from build123d import *

# Parameters (mm, degrees)
SKETCH_W             = 27
SKETCH_H             = 75
PAD_DEPTH            = 8
PAD001_DEPTH         = 2
SKETCH004_R          = 2.5
PAD002_DEPTH         = 2.2
SKETCH005_R          = 1.25
POCKET_DEPTH         = 4.201
SKETCH006_R          = 1.8
POCKET001_DEPTH      = 1.5
POCKET002_DEPTH      = 3.5
SKETCH008_R          = 2.5
PAD003_DEPTH         = 10
SKETCH009_R          = 1.5
POCKET003_DEPTH      = 13
POCKET004_DEPTH      = 1.4
POCKET004_DEPTH_BACK = 2
POCKET005_DEPTH      = 2


with BuildPart() as part:
    # Sketch → Pad (new body)
    with BuildSketch(Plane.XY):
        Polygon((0, 0), (15.5, 0), (15.5, 39.5), (15.5, 79), (0, 79), (-15.5, 79), (-15.5, 39.5), (-15.5, 0), align=None)
        with Locations((0, 39.5)):
            Rectangle(SKETCH_W, SKETCH_H, mode=Mode.SUBTRACT)
    extrude(amount=PAD_DEPTH)

    # Sketch001 → Pad001 (join)
    with BuildSketch(Plane.XY):
        Polygon((-15.5, 79), (-15.5, 39.5), (-15.5, 0), (0, 0), (15.5, 0), (15.5, 39.5), (15.5, 79), (0, 79), align=None)
    extrude(amount=-PAD001_DEPTH)

    # Sketch004 → Pad002 (join)
    with BuildSketch(Plane.XY):
        with Locations((-5.5, 69.25)):
            Circle(SKETCH004_R)
        with Locations((5.5, 69.25)):
            Circle(SKETCH004_R)
    extrude(amount=PAD002_DEPTH)

    # Sketch005 (on DatumPlane) → Pocket (cut, through all)
    with BuildSketch(Plane(origin=(-3, 69.25, 2.2), x_dir=(-1, 0, 0), z_dir=(0, 0, 1))):
        with Locations((2.5, 0)):
            Circle(SKETCH005_R)
        with Locations((-8.5, 0)):
            Circle(SKETCH005_R)
    extrude(amount=-POCKET_DEPTH, mode=Mode.SUBTRACT)

    # Sketch006 (on DatumPlane) → Pocket001 (cut)
    with BuildSketch(Plane(origin=(0, 79, -2), x_dir=(1, 0, 0), z_dir=(0, 0, -1))):
        with Locations((-5.5, 9.75)):
            Circle(SKETCH006_R)
        with Locations((5.5, 9.75)):
            Circle(SKETCH006_R)
    extrude(amount=-POCKET001_DEPTH, mode=Mode.SUBTRACT)

    # Sketch007 (on DatumPlane) → Pocket002 (cut)
    with BuildSketch(Plane(origin=(0, 69.25, 3.45), x_dir=(0, 1, 0), z_dir=(0, 0, 1))):
        Polygon((9.75, 0), (9.75, 4.25), (7.75, 4.25), (7.75, -4.25), (9.75, -4.25), align=None)
    extrude(amount=POCKET002_DEPTH, mode=Mode.SUBTRACT)

    # Sketch008 (on DatumPlane) → Pad003 (join)
    with BuildSketch(Plane(origin=(0, 79, 8), x_dir=(-1, 0, 0), z_dir=(0, 0, 1))):
        with Locations((-13, 15)):
            Circle(SKETCH008_R)
        with Locations((13, 15)):
            Circle(SKETCH008_R)
        with Locations((-13, 64)):
            Circle(SKETCH008_R)
        with Locations((13, 64)):
            Circle(SKETCH008_R)
    extrude(amount=-PAD003_DEPTH)

    # Sketch009 (on DatumPlane) → Pocket003 (cut)
    with BuildSketch(Plane(origin=(0, 79, 8), x_dir=(-1, 0, 0), z_dir=(0, 0, 1))):
        with Locations((-13, 15)):
            Circle(SKETCH009_R)
        with Locations((13, 15)):
            Circle(SKETCH009_R)
        with Locations((-13, 64)):
            Circle(SKETCH009_R)
        with Locations((13, 64)):
            Circle(SKETCH009_R)
    extrude(amount=-POCKET003_DEPTH, mode=Mode.SUBTRACT)

    # Sketch010 (on DatumPlane) → Pocket004 (cut, two sides)
    with BuildSketch(Plane(origin=(0, 69.25, 3.45), x_dir=(0, 1, 0), z_dir=(0, 0, 1))) as pocket004_sk:
        Polygon((7.75, 0), (7.75, 10), (8.75, 10), (8.75, -10), (7.75, -10), align=None)
    extrude(amount=-POCKET004_DEPTH, mode=Mode.SUBTRACT)
    extrude(pocket004_sk.sketch, amount=POCKET004_DEPTH_BACK, mode=Mode.SUBTRACT)

    # Sketch011 (on DatumPlane) → Pocket005 (cut)
    with BuildSketch(Plane.XZ):
        Polygon((0, 0), (4, 0), (4, 2.6), (-4, 2.6), (-4, 0), align=None)
    extrude(amount=-POCKET005_DEPTH, mode=Mode.SUBTRACT)


solid = part.part
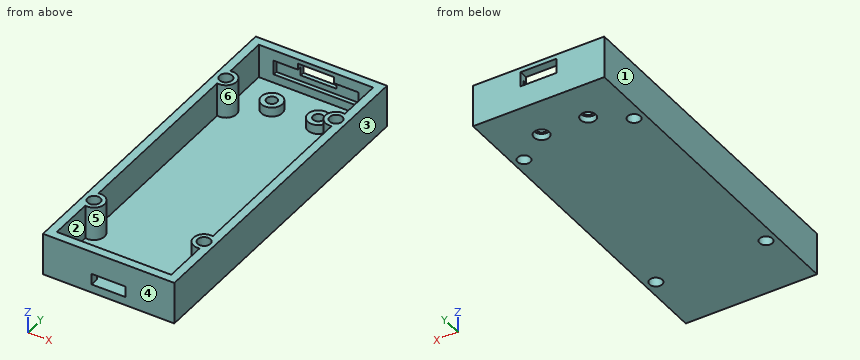
Work out the finished part from the listing and answer in its coordinate system (mm). Face numbers are marked on the shaded views. A direction names the side the tool comes from. Give positions to 0.01 mm unless a question says otherwise; leave off trailing zeros. Write each loop counter-clockwise with the first axis right and the second up, starting at its lowest first coordinate (ties: lowest second). Pieces come first, ordered by that corner, then holes.
Q1. A tool of negligible diameter and unlimited length cuts with its end or side. For the marked faces 1 and 2, from which of +Z, -Z, +X, -X, +Y, -Y can it reach the whole face along a straight path? Write none if from no direction.
Answer:
face 1: +Z, -Z, -X, +Y, -Y
face 2: +Z
Q2. The part is cut by section C-C on y = 69.25. State how many separate pieces and enclosed holes the cut face has, and give its area (3 significant figures).
Answer:
separate pieces: 3
enclosed holes: 0
area: 91.7 mm2
Q3. The part is cut by section D-D on x = -5.5. Give the vertices of the cut face in (y, z), and give its area (3 significant figures).
Answer:
outline: (0, -2) - (67.45, -2) - (67.45, -0.5) - (68, -0.5) - (68, 2.2) - (66.75, 2.2) - (66.75, 0) - (2, 0) - (2, 8) - (0, 8) - close; (70.5, -0.5) - (71.05, -0.5) - (71.05, -2) - (79, -2) - (79, 8) - (77, 8) - (77, 5.45) - (78, 5.45) - (78, 2.05) - (77, 2.05) - (77, 0) - (71.75, 0) - (71.75, 2.2) - (70.5, 2.2) - close
area: 185 mm2
Q4. For a pull along X with two mould halves and no side action, classify the marked faces 3, 4, 5 and 6 as released by +X, released by -X, zero draft, split by the parting line, or undercut.
Answer:
face 3: released by +X
face 4: zero draft
face 5: undercut
face 6: undercut
Q5. Straight lines are drawn through the part: L1, parallel to Y at x = 13, z = 3.25; L2, parallel to Y at x = -5.5, z = 0.95; L3, parallel to Y at x = 5.5, z = -1. For each, find the intervals that lie inside material, in ascending order.
Answer:
L1: y = 0 to 2, 12.5 to 13.5, 16.5 to 17.5, 61.5 to 62.5, 65.5 to 66.5, 77 to 79
L2: y = 0 to 2, 66.75 to 68, 70.5 to 71.75, 77 to 79
L3: y = 0 to 67.45, 71.05 to 79
Q6. The part is cut by section A-A on x = 2. Give the vertices of the cut face in (y, z), and give its area (3 significant figures).
Answer:
outline: (0, -2) - (79, -2) - (79, 3.45) - (78, 3.45) - (78, 2.05) - (77, 2.05) - (77, 0) - (0, 0) - close; (0, 2.6) - (2, 2.6) - (2, 8) - (0, 8) - close; (77, 6.95) - (79, 6.95) - (79, 8) - (77, 8) - close
area: 176 mm2
Q7. Given pin 1 (4 mm diameter, centred on x = 0, y = 11.5, fed in from +Z), flat-ended and moving along its own axis, determine where the tip first touches the part or whether it passes through.
Answer:
pin 1: stops at z = 0
Q8. The part is cut by section B-B on z = 4.5. Give the vertices of the cut face in (x, y).
Answer:
outline: (-15.5, 0) - (15.5, 0) - (15.5, 79) - (4.25, 79) - (4.25, 78) - (10, 78) - (10, 77) - (13.5, 77) - (13.5, 66.45) arc R2.5 ccw (long way) to (13.5, 61.55) - (13.5, 17.45) arc R2.5 ccw (long way) to (13.5, 12.55) - (13.5, 2) - (-13.5, 2) - (-13.5, 12.55) arc R2.5 ccw (long way) to (-13.5, 17.45) - (-13.5, 61.55) arc R2.5 ccw (long way) to (-13.5, 66.45) - (-13.5, 77) - (-10, 77) - (-10, 78) - (-4.25, 78) - (-4.25, 79) - (-15.5, 79) - close; hole circle Ø3 at (-13, 15); hole circle Ø3 at (-13, 64); hole circle Ø3 at (13, 15); hole circle Ø3 at (13, 64)
